```python
from build123d import *

# Parameters (mm, degrees)
F0_W      = 203.2
F0_H      = 249.9106
F0_R      = 2.794
F1_DEPTH  = 12.7
F2_R      = 4.0005
F3_DEPTH  = 12.701
F4_R      = 3.048
F5_DEPTH  = 12.701
F6_DEPTH  = 329
F7_R      = 7.1882
F8_DEPTH  = 4.064
F9_R      = 4.699
F10_DEPTH = 3.048
F11_R     = 5.461
F12_DEPTH = 3.81


# Not quite as in the source:
# - an extrude ends at something that could not be found from the text; its depth is read off the source's solid


with BuildPart() as f1:
    # F0 (on Front) → F1 (new body)
    with BuildSketch(Plane.XZ):
        Rectangle(F0_W, F0_H)
        with Locations((-11.938, 1.3843)):
            Circle(F0_R, mode=Mode.SUBTRACT)
        with Locations((-11.938, 37.3761)):
            Circle(F0_R, mode=Mode.SUBTRACT)
        with Locations((11.938, 1.3843)):
            Circle(F0_R, mode=Mode.SUBTRACT)
        with Locations((11.938, 37.3761)):
            Circle(F0_R, mode=Mode.SUBTRACT)
    extrude(amount=F1_DEPTH)

    # F2 (on face) → F3 (cut, through all)
    with BuildSketch(Plane.XZ.offset(12.7)):
        with Locations((-76.2, 115.4303)):
            Circle(F2_R)
        with Locations((-38.1, 115.4303)):
            Circle(F2_R)
        with Locations((0, 115.4303)):
            Circle(F2_R)
        with Locations((38.1, 115.4303)):
            Circle(F2_R)
        with Locations((76.2, 115.4303)):
            Circle(F2_R)
        with Locations((-76.2, -115.4303)):
            Circle(F2_R)
        with Locations((-38.1, -115.4303)):
            Circle(F2_R)
        with Locations((0, -115.4303)):
            Circle(F2_R)
        with Locations((38.1, -115.4303)):
            Circle(F2_R)
        with Locations((76.2, -115.4303)):
            Circle(F2_R)
    extrude(amount=-F3_DEPTH, mode=Mode.SUBTRACT)

    # F4 (on face) → F5 (cut, through all)
    with BuildSketch(Plane(origin=(0, 0, 0), x_dir=(-1, 0, 0), z_dir=(0, 1, 0))):
        with Locations((82.8548, -31.57982)):
            Circle(F4_R)
        with Locations((42.8498, -31.57982)):
            Circle(F4_R)
        with Locations((82.8548, -84.58962)):
            Circle(F4_R)
        with Locations((42.8498, -84.58962)):
            Circle(F4_R)
        with Locations((-42.8498, -31.57982)):
            Circle(F4_R)
        with Locations((-82.8548, -31.57982)):
            Circle(F4_R)
        with Locations((-82.8548, -84.58962)):
            Circle(F4_R)
        with Locations((-42.8498, -84.58962)):
            Circle(F4_R)
    extrude(amount=-F5_DEPTH, mode=Mode.SUBTRACT)

    # F0 (on Front) → F6 (cut, through all)
    with BuildSketch(Plane.XZ):
        Rectangle(F0_W, F0_H)
        with Locations((-11.938, 1.3843)):
            Circle(F0_R, mode=Mode.SUBTRACT)
        with Locations((-11.938, 37.3761)):
            Circle(F0_R, mode=Mode.SUBTRACT)
        with Locations((11.938, 1.3843)):
            Circle(F0_R, mode=Mode.SUBTRACT)
        with Locations((11.938, 37.3761)):
            Circle(F0_R, mode=Mode.SUBTRACT)
    extrude(amount=-F6_DEPTH, mode=Mode.SUBTRACT)

    # F7 (on face) → F8 (cut)
    with BuildSketch(Plane.XZ.offset(12.7)):
        with Locations((-76.2, -115.4303)):
            Circle(F7_R)
        with Locations((-38.1, -115.4303)):
            Circle(F7_R)
        with Locations((0, -115.4303)):
            Circle(F7_R)
        with Locations((38.1, -115.4303)):
            Circle(F7_R)
        with Locations((76.2, -115.4303)):
            Circle(F7_R)
        with Locations((-76.2, 115.4303)):
            Circle(F7_R)
        with Locations((-38.1, 115.4303)):
            Circle(F7_R)
        with Locations((0, 115.4303)):
            Circle(F7_R)
        with Locations((38.1, 115.4303)):
            Circle(F7_R)
        with Locations((76.2, 115.4303)):
            Circle(F7_R)
    extrude(amount=-F8_DEPTH, mode=Mode.SUBTRACT)

    # F9 (on face) → F10 (cut)
    with BuildSketch(Plane.XZ.offset(12.7)):
        with Locations((-11.938, 37.3761)):
            Circle(F9_R)
        with Locations((11.938, 37.3761)):
            Circle(F9_R)
        with Locations((11.938, 1.3843)):
            Circle(F9_R)
        with Locations((-11.938, 1.3843)):
            Circle(F9_R)
    extrude(amount=-F10_DEPTH, mode=Mode.SUBTRACT)

    # F11 (on face) → F12 (cut)
    with BuildSketch(Plane.XZ.offset(12.7)):
        with Locations((-82.8548, -31.57982)):
            Circle(F11_R)
        with Locations((-42.8498, -31.57982)):
            Circle(F11_R)
        with Locations((42.8498, -31.57982)):
            Circle(F11_R)
        with Locations((82.8548, -31.57982)):
            Circle(F11_R)
        with Locations((82.8548, -84.58962)):
            Circle(F11_R)
        with Locations((42.8498, -84.58962)):
            Circle(F11_R)
        with Locations((-42.8498, -84.58962)):
            Circle(F11_R)
        with Locations((-82.8548, -84.58962)):
            Circle(F11_R)
    extrude(amount=-F12_DEPTH, mode=Mode.SUBTRACT)


solid = f1.part
```
Geometry check sheet. Reference: the model listing, model coordinates, mm. A direction names the side the tool comes from. Give positions to 0.01 mm unless a question says otherwise; leave off trailing zeros. Write each loop counter-clockwise with the first axis right and the second up, starting at its lowest first coordinate (ties: lowest second). Pieces come first, ordered by that corner, then holes.
1) Section check A-A, the plane x = 0. Record the boundary of the cut face in (y, z).
2) Material ranges on L1, parallel to X at y = -8, z = 37.5; L2, parallel to Z at x = 80.5, y = -8.25; L3, parallel to Z at x = 47.5, y = -10, recorded low to high.
3) Access from +Z, -Z, +X, -X, +Y, -Y to the whole of each face (thin tool, end or side, straight path). Record for faces 4 (the cylindrical face through (-10.436, -4.758, 39.732)), 5 (the flat face through (3, -8.636, -119)).
4) Release check for a two-part mould opening along X. For faces 1 (the flat face through (-1, -6, 124.955)), 2 (the flat face through (-101.6, -6, -2)), 3 (the cylindrical face through (32.396, -10.696, 111.056)) record: pulls with the +X half, pulls with the -X half, needs draft (parallel to the pull), parting line crosses it, or undercut.
5) Section check B-B, the plane y = -3. State how many separate pieces and enclosed holes the cut face has, and give its area (3 significant figures).
6) Gauge pin test, flat ends, axial feed: pin 1 (7 mm diameter, centred on x = -82.85, z = -31.58, fed in from -Y); pin 2 (7 mm diameter, centred on x = -74, z = 116.5, fed in from -Y); pin 3 (3.5 mm diameter, centred on x = 11.94, z = 1.38, fed in from -Y). Record the tip position at first contact, or that the pin passes through.
Computed:
1. outline: (-12.7, -124.96) - (0, -124.96) - (0, -119.43) - (-8.64, -119.43) - (-8.64, -122.62) - (-12.7, -122.62) - close; (-12.7, -108.24) - (-8.64, -108.24) - (-8.64, -111.43) - (0, -111.43) - (0, 111.43) - (-8.64, 111.43) - (-8.64, 108.24) - (-12.7, 108.24) - close; (-12.7, 122.62) - (-8.64, 122.62) - (-8.64, 119.43) - (0, 119.43) - (0, 124.96) - (-12.7, 124.96) - close
2. L1: x = -101.6 to -14.73, -9.15 to 9.15, 14.73 to 101.6
2. L2: z = -124.96 to -86.52, -82.65 to -33.52, -29.64 to 124.96
2. L3: z = -124.96 to -87.45, -81.73 to -34.44, -28.72 to 124.96
3. face 4: +Y, -Y
3. face 5: -Y
4. face 1: needs draft
4. face 2: pulls with the -X half
4. face 3: undercut
5. separate pieces: 1
5. enclosed holes: 22
5. area: 49,900 mm2
6. pin 1: stops at y = -8.89
6. pin 2: stops at y = -8.64
6. pin 3: passes through
